```python
from build123d import *

# Parameters (mm, degrees)
SKETCH1_R           = 33
BOSS_EXTRUDE2_DEPTH = 6.5
SKETCH4_R           = 3
CUT_EXTRUDE1_DEPTH  = 6.5
BOSS_EXTRUDE3_DEPTH = 30
SKETCH6_R           = 8.25
CUT_EXTRUDE2_DEPTH  = 30
SKETCH8_R           = 1.5
CUT_EXTRUDE3_DEPTH  = 10
CUT_EXTRUDE4_DEPTH  = 30
FILLET12_R          = 2
FILLET13_R          = 2
FILLET14_R          = 2
FILLET15_R          = 2


with BuildPart() as part:
    # Sketch1 → Boss-Extrude2 (new body)
    with BuildSketch(Plane(origin=(0, 0, 0), x_dir=(1, 0, 0), z_dir=(0, 1, 0))):
        with Locations(Location((0, 0, 0), (0, 0, 90))):
            Circle(SKETCH1_R)
    extrude(amount=BOSS_EXTRUDE2_DEPTH)

    # Sketch4 → Cut-Extrude1 (cut)
    with BuildSketch(Plane(origin=(0, 6.5, 0), x_dir=(1, 0, 0), z_dir=(0, 1, 0))):
        with Locations(Location((0, 25, 0), (0, 0, 270))):
            Circle(SKETCH4_R)
        with Locations(Location((0, -25, 0), (0, 0, 270))):
            Circle(SKETCH4_R)
    extrude(amount=-CUT_EXTRUDE1_DEPTH, mode=Mode.SUBTRACT)

    # Sketch5 → Boss-Extrude3 (add)
    with BuildSketch(Plane(origin=(0, 6.5, 0), x_dir=(1, 0, 0), z_dir=(0, 1, 0))):
        Polygon((15, 0), (0, 0), (-15, 0), (-15, -15), (15, -15), align=None)
        Polygon((-15, 0), (0, 0), (15, 0), (15, 15), (-15, 15), align=None)
    extrude(amount=BOSS_EXTRUDE3_DEPTH)

    # Sketch6 → Cut-Extrude2 (cut)
    with BuildSketch(Plane(origin=(15, 0, 0), x_dir=(0, 0, -1), z_dir=(1, 0, 0))):
        with Locations((0, 18.5)):
            Circle(SKETCH6_R)
    extrude(amount=-CUT_EXTRUDE2_DEPTH, mode=Mode.SUBTRACT)

    # Sketch8 → Cut-Extrude3 (cut)
    with BuildSketch(Plane(origin=(0, 36.5, 0), x_dir=(1, 0, 0), z_dir=(0, 1, 0))):
        with Locations(Location((0, 0, 0), (0, 0, 270))):
            Circle(SKETCH8_R)
    extrude(amount=-CUT_EXTRUDE3_DEPTH, mode=Mode.SUBTRACT)

    # Sketch9 → Cut-Extrude4 (cut)
    with BuildSketch(Plane.ZY.offset(15)):
        Polygon((3, 32.75), (0, 32.75), (-3, 32.75), (-3, 29.75), (3, 29.75), align=None)
    extrude(amount=-CUT_EXTRUDE4_DEPTH, mode=Mode.SUBTRACT)

    # Fillet12
    fillet12_edges = [part.edges().sort_by_distance(p)[0] for p in [
        (0, 36.5, -15),
    ]]
    fillet(fillet12_edges, radius=FILLET12_R)

    # Fillet13
    fillet13_edges = [part.edges().sort_by_distance(p)[0] for p in [
        (0, 36.5, 15),
    ]]
    fillet(fillet13_edges, radius=FILLET13_R)

    # Fillet14
    fillet14_edges = [part.edges().sort_by_distance(p)[0] for p in [
        (15, 20.5, -15),
        (15, 35.914213562, -14.414213562),
        (15, 20.5, 15),
        (15, 36.5, 0),
        (15, 35.914213562, 14.414213562),
    ]]
    fillet(fillet14_edges, radius=FILLET14_R)

    # Fillet15
    fillet15_edges = [part.edges().sort_by_distance(p)[0] for p in [
        (-15, 20.5, -15),
        (-15, 36.5, 0),
        (-15, 35.914213562, -14.414213562),
        (-15, 20.5, 15),
        (-15, 35.914213562, 14.414213562),
    ]]
    fillet(fillet15_edges, radius=FILLET15_R)


solid = part.part
```
Read the model definition and answer for the solid it produces. Units are mm, in the model's axes. A direction names the side the tool comes from. Coordinates: 2 decimals unless noted, no trailing zeros. Order: outer loops, then holes, each group sorted by start corner. A loop starts at its lowest first (then second) coordinate and runs counter-clockwise, first axis right, second up. Notation, with made-up numbers: (86, 58.25) - (99, 58.25) arc R32 ccw to (99, 86.25) - close; hole circle Ø6 at (38, 56.25). An arc over 180 degrees is marked (long way). Answer as a JSON object with one key per item and string values. Group by question number.
Item 1: A tool of negligible diameter and unlimited length cuts with its end or side. For faces 4 (the face through (0.45, 34.65, 1.43)), 5 (the face through (0, 31, 3)), 6 (the face through (14.43, 20.3, 14.4)), 7 (the face through (14.43, 20.7, -14.4)), 8 (the face through (-14.43, 20.7, -14.4)), from which of +Z, -Z, +X, -X, +Y, -Y can it reach the whole face along a straight path? Write none if from no direction.
Item 2: Flat-ended cylindrical pins translate along their axes: P1, Ø12, axis at x = 21, y = 7, coming from the -Z side; P2, Ø2, axis at x = 24.5, y = 6, coming from the -Z side; P3, Ø2.5, axis at x = 0, z = 0, coming from the +Y side; P4, Ø15, axis at y = 18.5, z = 0, coming from the +X side. Find the tip coordinate at first contact, or state that the pin passes through.
Item 3: Consider probe 1 along X at (y, z) = (34.15, 0); probe 2 along Z at (x, y) = (4, 32.5); probe 3 along X at (y, z) = (18.5, -9). Determine where each line is inside the solid, lowest interval first. Write a range as from..to.
Item 4: Section B-B (z = 0) is taken. Give the vertices of the cut face in (x, y), plus the area to 3 significant figures.
Item 5: Section D-D (y = 7.5) is taken. Give the vertices of the cut face in (x, z), plus the area to 3 significant figures.
Item 6: The mould has two halves that part along Y. Classify faces 1 (the face through (0, 31, -3)), 2 (the face through (-0.18, 35.9, -14.43)), 3 (the face through (0, 20, 15)): +Y half, -Y half, draft (parallel to the pull), parting line (faces both ways), or undercut.
Item 7: Section A-A (x = 0) is taken. State how many separate pieces and enclosed holes the cut face has, plus the area to 3 significant figures.
Item 8: Section C-C (z = 25) is taken. Give the vertices of the cut face in (x, y).
Results are:
{
 "1": {"face 4": "+Y", "face 5": "+X, -X", "face 6": "+Z, +X, +Y", "face 7": "-Z, +X, +Y", "face 8": "-Z, -X, +Y"},
 "2": {"P1": "stops at z = -29.38", "P2": "stops at z = -23.17", "P3": "stops at y = 10.35", "P4": "passes through"},
 "3": {"probe 1": "x = -15..-1.5, 1.5..15", "probe 2": "z = -15..-3, 3..15", "probe 3": "x = -15..15"},
 "4": {"outline": "(-33, 0) - (33, 0) - (33, 6.5) - (15, 6.5) - (15, 10.25) - (-15, 10.25) - (-15, 6.5) - (-33, 6.5) - close; (-15, 26.75) - (-1.5, 26.75) - (-1.5, 29.75) - (-15, 29.75) - close; (-15, 32.75) - (-1.5, 32.75) - (-1.5, 36.5) - (-13, 36.5) arc R2 ccw to (-15, 34.5) - close; (1.5, 26.75) - (15, 26.75) - (15, 29.75) - (1.5, 29.75) - close; (1.5, 32.75) - (15, 32.75) - (15, 34.5) arc R2 ccw to (13, 36.5) - (1.5, 36.5) - close", "area": "722 mm^2"},
 "5": {"outline": "(-15, -13) arc R2 ccw to (-13, -15) - (13, -15) arc R2 ccw to (15, -13) - (15, 13) arc R2 ccw to (13, 15) - (-13, 15) arc R2 ccw to (-15, 13) - close", "area": "897 mm^2"},
 "6": {"face 1": "undercut", "face 2": "+Y half", "face 3": "draft"},
 "7": {"separate pieces": "3", "enclosed holes": "0", "area": "997 mm^2"},
 "8": {"outline": "(-21.54, 0) - (-3, 0) - (-3, 6.5) - (-21.54, 6.5) - close; (3, 0) - (21.54, 0) - (21.54, 6.5) - (3, 6.5) - close"}
}
